Drawing for the job (mm, zero at the part's lowest x, y, z). A direction names the side the tool comes from. Round coordinates to 2 decimals unless told otherwise and drop trailing zeros. Loops run counter-clockwise (first coordinate to the right, second up) from the corner with the lowest first, then second, coordinate; pieces in that order, holes last. Notation, with made-up numbers: (63.5, 58.5) -> (111.5, 58.5) arc R21 cw to (111.5, 90.5) -> close; hole circle Ø9 at (78.25, 52.25). An arc over 180 degrees is marked (long way). Put each result on its own line as item: value. Start each with the question number.
Item 1: Tool access for the marked faces 1, 2, 3, 4 and 5: list every direction of +Z, -Z, +X, -X, +Y, -Y with a clear straight run to the whole face (end or side of a thin tool).
Item 2: Cut at A-A, the plane y = 35.5. List the corners of the cut face in (x, z), plus the area to 3 significant figures.
Item 3: Pull direction Z, two halves, no side cores. Call the marked faces 6, 7, 8 and 9: +Z half, -Z half, draft (parallel to the pull), parting line (faces both ways), or undercut.
Item 4: Cut at C-C, the plane x = 34. List the corners of the cut face in (y, z), plus the area to 3 significant figures.
Item 5: Drill centre lines: probe 1 along Z at (x, y) = (24, 32.5); probe 2 along Z at (x, y) = (17.5, 30); probe 3 along X at (y, z) = (7, 28.5). Where is each one in solid material? Low to high. Write a range as [from, to].
Item 6: Cut at D-D, the plane y = 58. List the corners of the cut face in (x, z).
Item 7: Cut at B-B, the plane z = 61.5. List the corners of the cut face in (x, y), plus the area to 3 significant figures.
Item 8: Flat gauge pins, fed straight in: pin 1 Ø2 at (x, z) = (46, 63) entering from -Y; pin 2 Ø16 at (x, z) = (23.5, 25.5) entering from +Y; pin 3 Ø15 at (x, y) = (35, 22.5) entering from -Z; pin 4 Ø10 at (x, y) = (23.5, 9.5) entering from +Z. Where does each tip first touch, or does it go through?
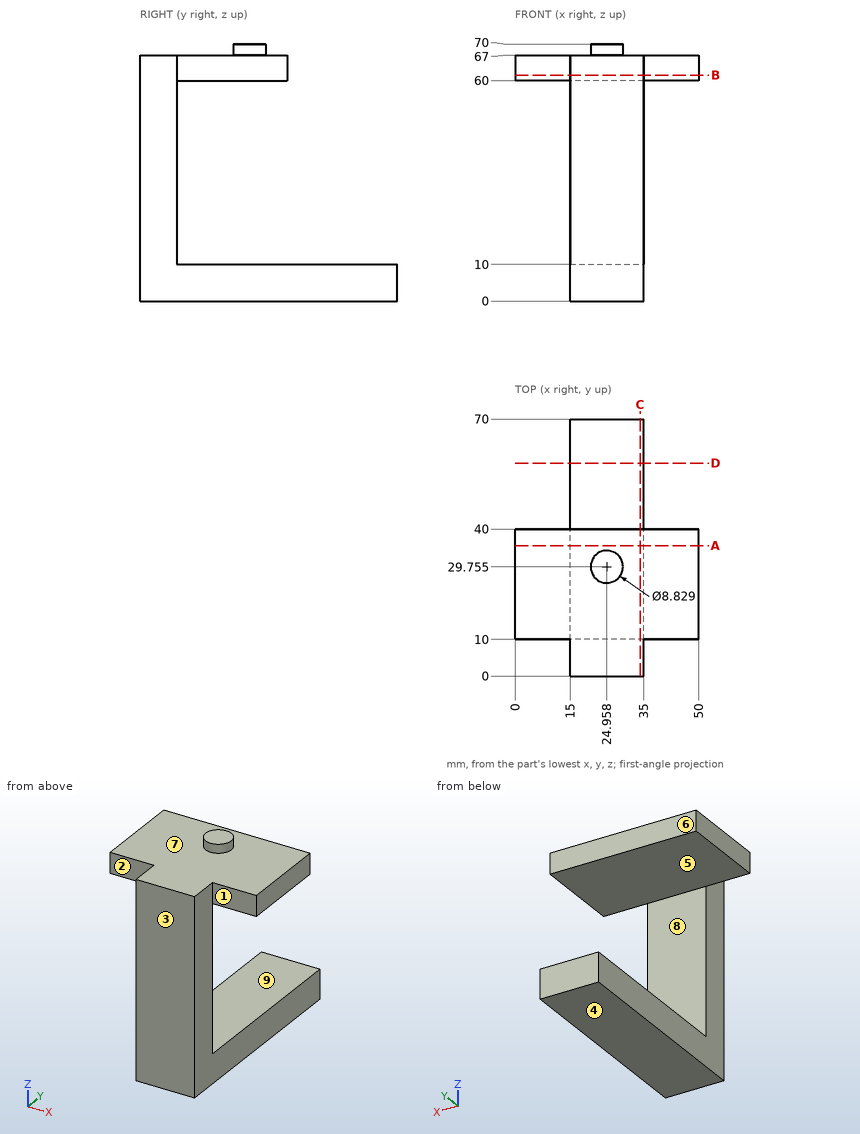
Reply:
1. face 1: +Z, -Z, +X, -Y
1. face 2: +Z, -Z, -X, -Y
1. face 3: +Z, -Z, +X, -X, -Y
1. face 4: -Z, +X, -X, +Y, -Y
1. face 5: +X, -X, +Y
2. outline: (0, 60) -> (50, 60) -> (50, 67) -> (0, 67) -> close; (15, 0) -> (35, 0) -> (35, 10) -> (15, 10) -> close
2. area: 550 mm^2
3. face 6: draft
3. face 7: +Z half
3. face 8: undercut
3. face 9: undercut
4. outline: (0, 0) -> (70, 0) -> (70, 10) -> (10, 10) -> (10, 60) -> (40, 60) -> (40, 67) -> (0, 67) -> close
4. area: 1,480 mm^2
5. probe 1: z = [0, 10], [60, 70]
5. probe 2: z = [0, 10], [60, 67]
5. probe 3: x = [15, 35]
6. outline: (15, 0) -> (35, 0) -> (35, 10) -> (15, 10) -> close
7. outline: (0, 10) -> (15, 10) -> (15, 0) -> (35, 0) -> (35, 10) -> (50, 10) -> (50, 40) -> (0, 40) -> close
7. area: 1,700 mm^2
8. pin 1: stops at y = 10
8. pin 2: stops at y = 10
8. pin 3: stops at z = 0
8. pin 4: stops at z = 67
